Design review of the part built by this model. Coordinates are the model's own, in mm. Face numbers are marked on the shaded views. Round coordinates to 2 decimals unless told otherwise and drop trailing zeros. Order: outer loops, then holes, each group sorted by start corner. A loop starts at its lowest first (then second) coordinate and runs counter-clockwise, first axis right, second up. Notation, with made-up numbers: M -36.5,4.5 L -8.5,4.5 A27 cw -8.5,28.5 Z; hole C 72.25,65.25 d8. An arc over 180 degrees is marked long. Write each question's results on one line, items separated by ' | '. Start each with the question number.
Item 1: Wall thickness on line 1 (Y direction, x = 137.75, z = 19.5); line 2 (X direction, y = 201.25, z = 19.75); line 3 (X direction, y = 202, z = 19.5): over which ranges is each line inside the solid? List them lowest first. Write a range as [from, to].
Item 2: Take a section at B-B, the plane z = 24.5. Write out the cut boundary in (x, y), plus the area to 3 significant figures.
Item 3: Clearance check with a flat-ended pin moving along its axis: pin 1 (3 mm diameter, centred on x = 133, z = 24, fed in from +Y). State where the tip first meets the part, or that it passes through.
Item 4: The part is to be moulded in two halves that separate along Y. For the marked faces 1, 2 and 3, say which applies: +Y half, -Y half, draft (parallel to the pull), parting line (faces both ways), or undercut.
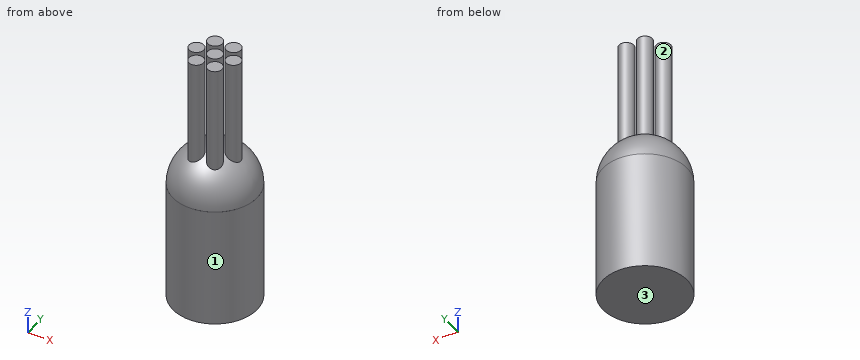
```python
from build123d import *

# Parameters (mm, degrees)
CYLINDER062_R     = 0.79375
CYLINDER062_DEPTH = 28
ARRAY003_COUNT    = 6
CYLINDER063_R     = 0.79375
CYLINDER063_DEPTH = 28
CYLINDER061_R     = 4.564063
CYLINDER061_DEPTH = 13


with BuildPart() as array003:
    # Cylinder062 → Cylinder062 (new body)
    with BuildSketch(Plane(origin=(2, 0, 0), x_dir=(1, 0, 0), z_dir=(0, 0, 1))):
        Circle(CYLINDER062_R)
    extrude(amount=CYLINDER062_DEPTH)

    # Array003: Array003 ×6 about axis
    array003_axis = Axis((0, 0, 0), (0, 0, 1))


with BuildPart() as array003_1:
    add(array003.part)
    for i in range(1, ARRAY003_COUNT):
        add(array003.part.rotate(array003_axis, i * 360 / ARRAY003_COUNT))


with BuildPart() as obj1:
    # Cylinder063 → Cylinder063 (new body)
    with BuildSketch(Plane.XY):
        Circle(CYLINDER063_R)
    extrude(amount=CYLINDER063_DEPTH)

    # Fusion026: union Array003
    add(array003_1.part)


with BuildPart() as compression002:
    # Sphere002 → Sphere002 (revolve)
    with BuildSketch(Plane(origin=(0, 0, 13), x_dir=(1, 0, 0), z_dir=(0, -1, 0))):
        with BuildLine():
            ThreePointArc((0, -4.56), (4.56, 0), (0, 4.56))
            Line((0, 4.56), (0, -4.56))
        make_face()
    revolve(axis=Axis((0, 0, 13), (0, 0, 1)))


with BuildPart() as obj2:
    # Cylinder061 → Cylinder061 (new body)
    with BuildSketch(Plane.XY):
        Circle(CYLINDER061_R)
    extrude(amount=CYLINDER061_DEPTH)

    # Fusion027: union obj1, Compression002
    add(obj1.part)
    add(compression002.part)


with BuildPart() as obj2_1:
    # Fusion027 placement: moved
    add(obj2.part.moved(Location((136.75, 199.75, 0))))


solid = obj2_1.part
```
Results list:
1) line 1: [197.22, 198.81], [200.69, 202.28] | line 2: [134.99, 136.51], [136.99, 138.51] | line 3: [135.15, 136.35], [137.15, 138.35]
2) outline: C 134.75,199.75 d1.59; C 135.75,198.02 d1.59; C 135.75,201.48 d1.59; C 136.75,199.75 d1.59; C 137.75,198.02 d1.59; C 137.75,201.48 d1.59; C 138.75,199.75 d1.59 | area: 13.9 mm²
3) pin 1: y = 200.5
4) face 1: parting line | face 2: undercut | face 3: draft
